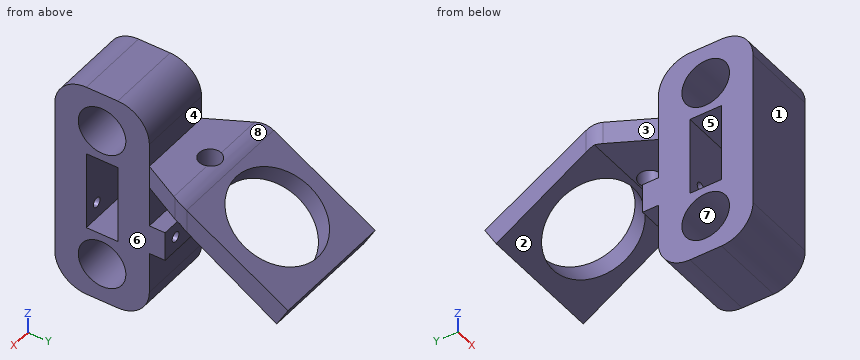
```python
from build123d import *

# Parameters (mm, degrees)
SKETCH_1_W          = 24
SKETCH_1_H          = 70
EXTRUDE_1_DEPTH     = 30
SKETCH_2_R          = 7.55
CUT_EXTRUDE_1_DEPTH = 71.806439045
SKETCH_3_W          = 25
SKETCH_3_H          = 10
CUT_EXTRUDE_2_DEPTH = 71.806439045
SKETCH_4_W          = 24
SKETCH_4_H          = 9.317438099
EXTRUDE_2_DEPTH     = 5
SKETCH_5_R          = 1.55
CUT_EXTRUDE_3_DEPTH = 31
FILLET_1_R          = 10
SKETCH_6_W          = 24
SKETCH_6_H          = 7.198600856
EXTRUDE_3_DEPTH     = 15
EXTRUDE_4_DEPTH     = 24
EXTRUDE_5_DEPTH     = 8
EXTRUDE_6_DEPTH     = 8
SKETCH_10_R         = 15
CUT_EXTRUDE_4_DEPTH = 16
EXTRUDE_7_DEPTH     = 7.198600855
EXTRUDE_8_DEPTH     = 7.198600855
FILLET_2_R          = 10
FILLET_3_R          = 10
SKETCH_14_R         = 3.5
CUT_EXTRUDE_5_DEPTH = 13


with BuildPart() as part:
    # 草图1 → 凸台-拉伸1 (new body)
    with BuildSketch(Plane(origin=(0, 0, 0), x_dir=(1, 0, 0), z_dir=(0, 1, 0))):
        with Locations((20.241900648, -24.477321814)):
            Rectangle(SKETCH_1_W, SKETCH_1_H)
    extrude(amount=EXTRUDE_1_DEPTH)

    # 草图2 → 切除-拉伸1 (cut, through all)
    with BuildSketch(Plane(origin=(32.241900648, 0, 0), x_dir=(0, 0, -1), z_dir=(1, 0, 0))):
        with Locations((-46.977321814, 15)):
            Circle(SKETCH_2_R)
        with Locations((-1.977321814, 15)):
            Circle(SKETCH_2_R)
    extrude(amount=-CUT_EXTRUDE_1_DEPTH, mode=Mode.SUBTRACT)

    # 草图3 → 切除-拉伸2 (cut, through all)
    with BuildSketch(Plane(origin=(32.241900648, 0, 0), x_dir=(0, 0, -1), z_dir=(1, 0, 0))):
        with Locations((-24.477321814, 15)):
            Rectangle(SKETCH_3_W, SKETCH_3_H)
    extrude(amount=-CUT_EXTRUDE_2_DEPTH, mode=Mode.SUBTRACT)

    # 草图4 → 凸台-拉伸2 (add)
    with BuildSketch(Plane(origin=(0, 30, 0), x_dir=(1, 0, 0), z_dir=(0, 1, 0))):
        with Locations((20.241900648, -17.269567559)):
            Rectangle(SKETCH_4_W, SKETCH_4_H)
    extrude(amount=EXTRUDE_2_DEPTH)

    # 草图5 → 切除-拉伸3 (cut)
    with BuildSketch(Plane(origin=(0, 35, 0), x_dir=(1, 0, 0), z_dir=(0, 1, 0))):
        with Locations(Location((27.441174565, -17.269567558, 0), (0, 0, 270))):
            Circle(SKETCH_5_R)
        with Locations(Location((13.141174565, -17.269567558, 0), (0, 0, 270))):
            Circle(SKETCH_5_R)
    extrude(amount=-CUT_EXTRUDE_3_DEPTH, mode=Mode.SUBTRACT)

    # 圆角1
    fillet_1_edges = [part.edges().sort_by_distance(p)[0] for p in [
        (20.241900648, 30, -10.522678186),
        (20.241900648, 0, -10.522678186),
        (20.241900648, 0, 59.477321814),
        (20.241900648, 30, 59.477321814),
    ]]
    fillet(fillet_1_edges, radius=FILLET_1_R)

    # 草图6 → 凸台-拉伸3 (add)
    with BuildSketch(Plane(origin=(0, 30, 0), x_dir=(1, 0, 0), z_dir=(0, 1, 0))):
        with Locations((20.241900648, -38.481509693)):
            Rectangle(SKETCH_6_W, SKETCH_6_H)
    extrude(amount=EXTRUDE_3_DEPTH)

    # 草图7 → 凸台-拉伸4 (add)
    with BuildSketch(Plane.ZY.offset(-8.241900648)):
        Polygon((42.080810121, 45), (21.912574503, 79.54333904), (15.694773475, 75.913056629), (34.882209265, 45), align=None)
    extrude(amount=-EXTRUDE_4_DEPTH)

    # 草图8 → 凸台-拉伸5 (add)
    with BuildSketch(Plane.ZY.offset(-8.241900648)):
        Polygon((42.080810121, 45), (34.882209265, 45), (15.694773475, 75.913056629), (21.912574503, 79.54333904), align=None)
    extrude(amount=EXTRUDE_5_DEPTH)

    # 草图9 → 凸台-拉伸6 (add)
    with BuildSketch(Plane(origin=(32.241900648, 0, 0), x_dir=(0, 0, -1), z_dir=(1, 0, 0))):
        Polygon((-42.080810121, 45), (-34.882209265, 45), (-15.694773475, 75.913056629), (-21.912574503, 79.54333904), align=None)
    extrude(amount=EXTRUDE_6_DEPTH)

    # 草图10 → 切除-拉伸4 (cut)
    with BuildSketch(Plane(origin=(0, 29.763050525, 50.976950321), x_dir=(1, 0, 0), z_dir=(0, 0.5042058904481267, 0.8635834760099408))):
        with Locations(Location((20.241900648, 37.643864083, 0), (0, 0, 270))):
            Circle(SKETCH_10_R)
    extrude(amount=-CUT_EXTRUDE_4_DEPTH, mode=Mode.SUBTRACT)

    # 草图12 → 凸台-拉伸7 (add)
    with BuildSketch(Plane.XY.offset(42.080810121)):
        Polygon((0.241900648, 45), (8.241900648, 45), (8.241900648, 30), align=None)
    extrude(amount=-EXTRUDE_7_DEPTH)

    # 草图13 → 凸台-拉伸8 (add)
    with BuildSketch(Plane.XY.offset(42.080810121)):
        Polygon((40.241900648, 45), (32.241900648, 45), (32.241900648, 30), align=None)
    extrude(amount=-EXTRUDE_8_DEPTH)

    # 圆角2
    fillet_2_edges = [part.edges().sort_by_distance(p)[0] for p in [
        (20.241900648, 45, 42.080810121),
    ]]
    fillet(fillet_2_edges, radius=FILLET_2_R)

    # 圆角3
    fillet_3_edges = [part.edges().sort_by_distance(p)[0] for p in [
        (0.241900648, 45, 38.295029227),
        (40.241900648, 45, 38.295029227),
    ]]
    fillet(fillet_3_edges, radius=FILLET_3_R)

    # 草图14 → 切除-拉伸5 (cut)
    with BuildSketch(Plane.XY.offset(42.080810121)):
        with Locations((20.241537607, 41)):
            Circle(SKETCH_14_R)
    extrude(amount=-CUT_EXTRUDE_5_DEPTH, mode=Mode.SUBTRACT)


solid = part.part
```
CAD build for the part. Positions are in the model's coordinates, mm. Face numbers are marked on the shaded views. A direction names the side the tool comes from. Give positions to 0.01 mm unless a question says otherwise; leave off trailing zeros. Write each loop counter-clockwise with the first axis right and the second up, starting at its lowest first coordinate (ties: lowest second). Pieces come first, ordered by that corner, then holes. Notation, with made-up numbers: (87.25, 51) -> (96.25, 51) arc R21 cw to (96.25, 68) -> close; hole circle Ø10 at (-11, -11). An arc over 180 degrees is marked (long way). Write each question's results on one line, items separated by ' | '.
1. Which spindle directions (+Z, -Z, +X, -X, +Y, -Y) get a long thin tool onto all of the face, cutting with end or side? Do the marked faces 1, 2, 3, 4 and 5. Say none if no direction does.
Geometry check:
face 1: +Z, -Z, +X, -X, -Y | face 2: -Z, +X, -X | face 3: +Z, -Z, -X, -Y | face 4: +Z, +X, -X, +Y | face 5: +X, -X
2. Two-plate mould, pull along Y, no slides. Class the marked faces 6, 7 and 8: pulls with the +Y half, pulls with the -Y half, needs draft (parallel to the pull), parting line crosses it, or undercut.
Geometry check:
face 6: needs draft | face 7: undercut | face 8: pulls with the +Y half
3. Drop flat-ended pins along their axis: P1, Ø14.5, axis at x = 22.5, z = 5, coming from the +Y side; P2, Ø2, axis at x = 18.5, y = 23.5, coming from the -Z side; P3, Ø13.5, axis at x = 21.5, y = 38.5, coming from the +Z side; P4, Ø9, axis at y = 15, z = 46.98, coming from the +X side (1 decimal). Give the stop position or say it passes through.
Geometry check:
P1: y = 30 | P2: z = -10.21 | P3: z = 42.08 | P4: through
4. Cut at C-C, the plane y = 41. Write the cut outline in (x, z).
Geometry check:
outline: (2.38, 34.88) -> (16.74, 34.88) -> (16.74, 42.08) -> (2.38, 42.08) -> close; (23.74, 34.88) -> (38.11, 34.88) -> (38.11, 42.08) -> (23.74, 42.08) -> close
5. Cut at B-B, the plane z = 48. Write the cut outline in (x, y), then the cut area to 3 significant figures.
Geometry check:
outline: (8.24, 0) -> (32.24, 0) -> (32.24, 7.52) -> (8.24, 7.52) -> close; (8.24, 22.48) -> (32.24, 22.48) -> (32.24, 30) -> (8.24, 30) -> close | area: 361 mm²
6. Cut at D-D, the plane y = 6. Write the cut outline in (x, z).
Geometry check:
outline: (8.24, -9.69) -> (32.24, -9.69) -> (32.24, 58.64) -> (8.24, 58.64) -> close; hole circle Ø3.1 at (13.14, 17.27); hole circle Ø3.1 at (27.44, 17.27)
7. Cut at A-A, the plane y = 15. Write the cut outline in (x, z).
Geometry check:
outline: (8.24, -10.52) -> (32.24, -10.52) -> (32.24, -5.57) -> (8.24, -5.57) -> close; (8.24, 9.53) -> (32.24, 9.53) -> (32.24, 11.98) -> (8.24, 11.98) -> close; (8.24, 36.98) -> (32.24, 36.98) -> (32.24, 39.43) -> (8.24, 39.43) -> close; (8.24, 54.53) -> (32.24, 54.53) -> (32.24, 59.48) -> (8.24, 59.48) -> close
8. Wall check: probe 1 along Z at (x, y) = (11, 16.5); probe 2 along X at (y, z) = (24, 46); probe 3 along Y at (x, z) = (30.5, 34.5). Give the ranges that are in metal, low to high. Write a range as [from, to].
Geometry check:
probe 1: [-10.52, -5.42], [9.38, 11.98], [36.98, 39.58], [54.38, 59.48] | probe 2: [8.24, 32.24] | probe 3: [0, 10], [20, 30], [45.62, 51.06]
